```python
from build123d import *

# Parameters (mm, degrees)
F1_DEPTH = 70
F2_DEPTH = 5
F4_DEPTH = 25
F5_DEPTH = 5
F6_DEPTH = 5
F7_DEPTH = 13.5


with BuildPart() as f1:
    # F0 (on Right) → F1 (new body)
    with BuildSketch(Plane.YZ):
        Polygon((0, 26.0990989228), (0, 0), (0, -10.9009010772), (8.5, -35.9009010772), (13.5, -35.9009010772), (13.5, -15.9009010772), (33.5, -15.9009010772), (33.5, -10.9009010772), (13.5, -10.9009010772), (13.5, -5.7190796932), (13.5, 8.0284756223), (13.5, 26.0990989228), align=None)
    extrude(amount=F1_DEPTH)

    # F2 (add): a face of the model
    f2_faces = [f1.faces().sort_by_distance(p)[0] for p in [
        (35, 6.75, 26.0990989228),
    ]]
    extrude(f2_faces, amount=F2_DEPTH)

    # F3 (on face) → F4 (cut)
    with BuildSketch(Plane(origin=(0, 13.5, 0), x_dir=(-1, 0, 0), z_dir=(0, 1, 0))):
        Polygon((-70, 37.3218916357), (-70, 31.0990989228), (-40, 31.0990989228), (-35, 31.0990989228), (-30, 31.0990989228), (0, 31.0990989228), (0, 37.3218916357), align=None)
        Polygon((-70, -6.9171057179), (-70, -10.9009010772), (0, -10.9009010772), (0, -6.9171057179), (0, 31.0990989228), (-30, 31.0990989228), (-35, 31.0990989228), (-40, 31.0990989228), (-70, 31.0990989228), align=None)
    extrude(amount=-F4_DEPTH, mode=Mode.SUBTRACT)

    # F5 (add): a face of the model
    f5_faces = [f1.faces().sort_by_distance(p)[0] for p in [
        (35, 33.5, -13.4009010772),
    ]]
    extrude(f5_faces, amount=F5_DEPTH)

    # F6 (add): a face of the model
    f6_faces = [f1.faces().sort_by_distance(p)[0] for p in [
        (35, 11, -35.9009010772),
    ]]
    extrude(f6_faces, amount=F6_DEPTH)

    # F3 (on face) → F7 (join)
    with BuildSketch(Plane(origin=(0, 13.5, 0), x_dir=(-1, 0, 0), z_dir=(0, 1, 0))):
        Polygon((-70, -6.9171057179), (-70, -10.9009010772), (0, -10.9009010772), (0, -6.9171057179), (0, 37.3218916357), (-70, 37.3218916357), (-70, 31.0990989228), align=None)
    extrude(amount=-F7_DEPTH)


solid = f1.part
```
Design review of the part built by this model. Coordinates are the model's own, in mm. A direction names the side the tool comes from. Round coordinates to 2 decimals unless told otherwise and drop trailing zeros. Write each loop counter-clockwise with the first axis right and the second up, starting at its lowest first coordinate (ties: lowest second). Pieces come first, ordered by that corner, then holes.
Item 1: We need section A-A on x = 8.5. Write out the cut boundary in (y, z).
Item 2: For probe 1 along Y at (x, z) = (15, 13.5); probe 2 along Z at (x, y) = (65, 20); probe 3 along Y at (x, z) = (28.5, -30), list the stretches that pass through material, from the lowest coordinate up.
Item 3: For faces 1 (the flat face through (35, 8.5, -38)), 2 (the flat face through (35, 13.5, -28)), 3 (the flat face through (35, 26, -10.901)), list the 3-axis set-ups (+Z, -Z, +X, -X, +Y, -Y) from which the entire face can be reached by the end or side of a thin tool; tool diameter is ignored.
Item 4: We need section C-C on y = 19. Write out the cut boundary in (x, z).
Item 5: Clearance check with flat-ended pins moving along their axes: pin 1 Ø2 at (y, z) = (9.5, -16) entering from -X; pin 2 Ø5 at (x, z) = (40, -25) entering from +Y; pin 3 Ø12.5 at (x, y) = (37.5, 27.5) entering from +Z; pin 4 Ø10 at (x, y) = (37.5, 23) entering from -Z. State where each tip first meets the part, or that it passes through.
Item 6: We need section B-B on z = 7.5. Write out the cut boundary in (x, y), and give its area (3 significant figures).
Returned:
1. outline: (0, -10.9) - (8.5, -35.9) - (8.5, -40.9) - (13.5, -40.9) - (13.5, -15.9) - (38.5, -15.9) - (38.5, -10.9) - (13.5, -10.9) - (13.5, 37.32) - (0, 37.32) - close
2. probe 1: y = 0 to 13.5
2. probe 2: z = -15.9 to -10.9
2. probe 3: y = 6.49 to 13.5
3. face 1: -Z, +X, -X, -Y
3. face 2: -Z, +X, -X, +Y
3. face 3: +Z, +X, -X, +Y
4. outline: (0, -15.9) - (70, -15.9) - (70, -10.9) - (0, -10.9) - close
5. pin 1: stops at x = 0
5. pin 2: stops at y = 13.5
5. pin 3: stops at z = -10.9
5. pin 4: stops at z = -15.9
6. outline: (0, 0) - (70, 0) - (70, 13.5) - (0, 13.5) - close
6. area: 945 mm2
